Verification items for the finished model (mm, model axes). Face numbers are marked on the shaded views. A direction names the side the tool comes from. Coordinates: 2 decimals unless noted, no trailing zeros. Order: outer loops, then holes, each group sorted by start corner. A loop starts at its lowest first (then second) coordinate and runs counter-clockwise, first axis right, second up. Notation, with made-up numbers: M 54.5,-26 L 61.5,-26 A23 ccw 61.5,7 Z; hole C 9.25,72 d7. An arc over 180 degrees is marked long. Answer as a JSON object with one key per item and string values. Group by question number.
(1) Cross-section at A-A (x = 0). Enter the section's corners in (y, z).
(2) Cross-section at D-D (x = -21.5). Enter the section's corners in (y, z).
(3) Cross-section at C-C (z = 37.5). Enter the section's corners in (x, y).
(4) Mould release check, pull along Z, two halves, no side actions. Record for the marked faces 5, 6 and 7: released by +Z, released by -Z, zero draft, split by the parting line, or undercut.
(5) Access from +Z, -Z, +X, -X, +Y, -Y to the whole of each face (thin tool, end or side, straight path). Record for the marked faces 1, 2, 3 and 4.
(6) Material ranges on line 1 (Z direction, x = -3.5, y = 29.5); line 2 (Z direction, x = 19.5, y = -10.5); line 3 (X direction, y = 5, z = 56.5), recorded low to high.
(7) Gauge pin test, flat ends, axial feed: pin 1 Ø2 at (y, z) = (-1, 23.5) entering from -X; pin 2 Ø1.5 at (x, y) = (9.5, -7.5) entering from -Z; pin 3 Ø5 at (y, z) = (8.5, 21) entering from +X. Record the tip position at first contact, or that the pin passes through.
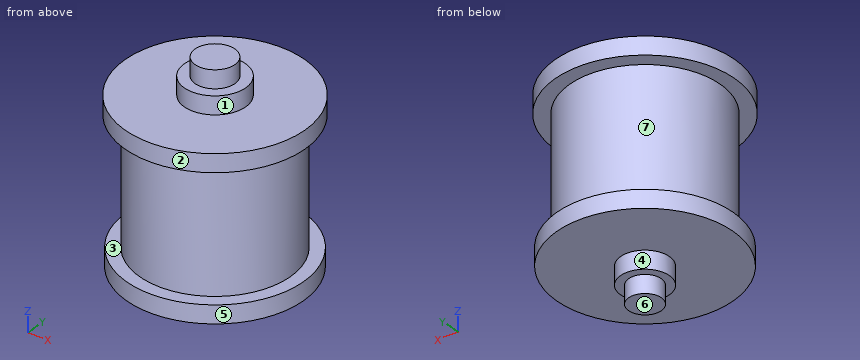
from build123d import *

# Parameters (mm, degrees)
SKETCH1_R           = 49.444265543
BOSS_EXTRUDE1_DEPTH = 10
SKETCH4_R           = 42.186355854
BOSS_EXTRUDE2_DEPTH = 70
SKETCH5_R           = 50.299469204
BOSS_EXTRUDE3_DEPTH = 10
SKETCH6_R           = 13.695749192
BOSS_EXTRUDE4_DEPTH = 10
SKETCH7_R           = 9.193746995
BOSS_EXTRUDE5_DEPTH = 10
SKETCH8_R           = 17.176734278
BOSS_EXTRUDE6_DEPTH = 10
SKETCH9_R           = 11.157494919
BOSS_EXTRUDE7_DEPTH = 10
SCALE1_SCALE        = 0.9
SCALE2_SCALE        = 0.7


with BuildPart() as part:
    # Sketch1 → Boss-Extrude1 (new body)
    with BuildSketch(Plane.XY):
        Circle(SKETCH1_R)
    extrude(amount=BOSS_EXTRUDE1_DEPTH)

    # Sketch4 → Boss-Extrude2 (add)
    with BuildSketch(Plane.XY.offset(10)):
        Circle(SKETCH4_R)
    extrude(amount=BOSS_EXTRUDE2_DEPTH)

    # Sketch5 → Boss-Extrude3 (add)
    with BuildSketch(Plane.XY.offset(80)):
        Circle(SKETCH5_R)
    extrude(amount=BOSS_EXTRUDE3_DEPTH)

    # Sketch6 → Boss-Extrude4 (add)
    with BuildSketch(Plane(origin=(0, 0, 0), x_dir=(-1, 0, 0), z_dir=(0, 0, -1))):
        Circle(SKETCH6_R)
    extrude(amount=BOSS_EXTRUDE4_DEPTH)

    # Sketch7 → Boss-Extrude5 (add)
    with BuildSketch(Plane(origin=(0, 0, -10), x_dir=(-1, 0, 0), z_dir=(0, 0, -1))):
        Circle(SKETCH7_R)
    extrude(amount=BOSS_EXTRUDE5_DEPTH)

    # Sketch8 → Boss-Extrude6 (add)
    with BuildSketch(Plane.XY.offset(90)):
        Circle(SKETCH8_R)
    extrude(amount=BOSS_EXTRUDE6_DEPTH)

    # Sketch9 → Boss-Extrude7 (add)
    with BuildSketch(Plane.XY.offset(100)):
        Circle(SKETCH9_R)
    extrude(amount=BOSS_EXTRUDE7_DEPTH)


with BuildPart() as part_1:
    # Scale1: scaled about (0, 0, 45.617034172)
    add(part.part.scale(SCALE1_SCALE).moved(Location((0, 0, 4.561703417))))


with BuildPart() as part_2:
    # Scale2: scaled about (0, 0, 45.617034172)
    add(part_1.part.scale(SCALE2_SCALE).moved(Location((0, 0, 13.685110252))))


solid = part_2.part
Taken from the geometry:
{
 "1": {"outline": "M -31.69,67.28 L -26.58,67.28 L -26.58,23.18 L -31.15,23.18 L -31.15,16.88 L -8.63,16.88 L -8.63,10.58 L -5.79,10.58 L -5.79,4.28 L 5.79,4.28 L 5.79,10.58 L 8.63,10.58 L 8.63,16.88 L 31.15,16.88 L 31.15,23.18 L 26.58,23.18 L 26.58,67.28 L 31.69,67.28 L 31.69,73.58 L 10.82,73.58 L 10.82,79.88 L 7.03,79.88 L 7.03,86.18 L -7.03,86.18 L -7.03,79.88 L -10.82,79.88 L -10.82,73.58 L -31.69,73.58 Z"},
 "2": {"outline": "M -23.28,67.28 L -15.62,67.28 L -15.62,23.18 L -22.54,23.18 L -22.54,16.88 L 22.54,16.88 L 22.54,23.18 L 15.62,23.18 L 15.62,67.28 L 23.28,67.28 L 23.28,73.58 L -23.28,73.58 Z"},
 "3": {"outline": "C 0,0 d53.15"},
 "4": {"face 5": "zero draft", "face 6": "released by -Z", "face 7": "undercut"},
 "5": {"face 1": "+Z", "face 2": "+Z, -Z", "face 3": "none", "face 4": "-Z"},
 "6": {"line 1": "z = 16.88 to 23.18, 67.28 to 73.58", "line 2": "z = 16.88 to 73.58", "line 3": "x = -26.1 to 26.1"},
 "7": {"pin 1": "stops at x = -31.15", "pin 2": "stops at z = 16.88", "pin 3": "stops at x = 30.57"}
}
